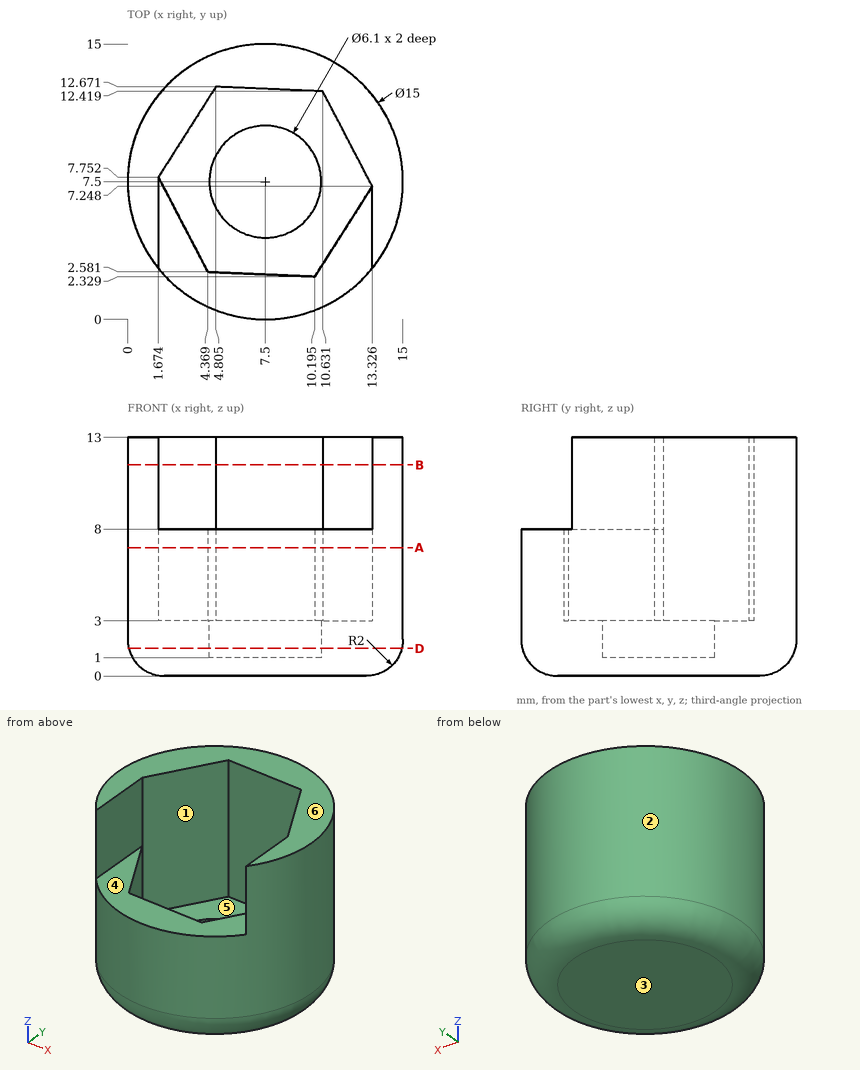
Could you check a few things on this drawing? It's one solid part, dimensions in mm from its lowest x, y, z. A direction names the side the tool comes from. Round coordinates to 2 decimals unless told otherwise and drop trailing zeros. Order: outer loops, then holes, each group sorted by start corner. A loop starts at its lowest first (then second) coordinate and runs counter-clockwise, first axis right, second up. Notation, with made-up numbers: M -29.75,44 L 12.25,44 A18 ccw 12.25,62 Z; hole C 75.5,24.25 d5. An arc over 180 degrees is marked long. Use a Markdown table: item, result.
1) On a 3-axis mill with a long thin cutter (end or side, diameter ignored), from which of +Z, -Z, +X, -X, +Y, -Y can I reach the whole of each face in a straight line? I mean the marked faces 4, 5 and 6. Say none if no direction works.
Geometry says:
| item | result |
|---|---|
| face 4 | +Z, -Y |
| face 5 | +Z |
| face 6 | +Z, +X, -X, +Y, -Y |
2) If I drill on line 1 along Y through (x, z) = (7.5, 1.95); line 2 along X through (y, z) = (5, 6.25) (1 decimal); line 3 along X through (y, z) = (9.75, 3.5) (1 decimal), over which ranges is the centre line in solid material (lowest first)?
Geometry says:
| item | result |
|---|---|
| line 1 | y = 0 to 4.45, 10.55 to 15 |
| line 2 | x = 0.4 to 3.1, 11.9 to 14.6 |
| line 3 | x = 0.3 to 2.9, 12 to 14.7 |
3) Imagine slicing it at D-D (z = 1.5). List the corners of the cut face in (x, y) for me.
Geometry says:
| item | result |
|---|---|
| outline | C 7.5,7.5 d14.87; hole C 7.5,7.5 d6.1 |
4) Imagine slicing it at A-A (z = 7). List the corners of the cut face in (x, y) for me (1 decimal).
Geometry says:
| item | result |
|---|---|
| outline | C 7.5,7.5 d15; hole M 1.7,7.8 L 4.4,2.6 L 10.2,2.3 L 13.3,7.2 L 10.6,12.4 L 4.8,12.7 Z |
5) I'm going to push flat-ended pins straight in: P1, Ø6, axis at x = 4, z = 3.5, coming from the +Y side; P2, Ø6.5, axis at x = 6.5, y = 9, coming from the +Z side; P3, Ø2, axis at y = 1.5, z = 6.5, coming from the -X side. Where does each tip first touch, or does it pass through?
Geometry says:
| item | result |
|---|---|
| P1 | stops at y = 14.98 |
| P2 | stops at z = 3 |
| P3 | stops at x = 1.91 |
6) Imagine slicing it at B-B (z = 11.5). List the corners of the cut face in (x, y) for me (1 decimal).
Geometry says:
| item | result |
|---|---|
| outline | M 1.7,2.8 L 1.7,7.8 L 4.8,12.7 L 10.6,12.4 L 13.3,7.2 L 13.3,2.8 A7.5 ccw long Z |
7) If we mould it in two halves opening along Y, with no side actions, what happens to the marked faces 1, 2 and 3? For each: +Y half, -Y half, draft (parallel to the pull), parting line (faces both ways), or undercut.
Geometry says:
| item | result |
|---|---|
| face 1 | undercut |
| face 2 | parting line |
| face 3 | draft |
